Here's how the part is built. I have some questions about the finished solid (model axes, mm). Coordinates: 2 decimals unless noted, no trailing zeros. Order: outer loops, then holes, each group sorted by start corner. A loop starts at its lowest first (then second) coordinate and runs counter-clockwise, first axis right, second up. Notation, with made-up numbers: (-12, 14.25) - (-6, 14.25) arc R31 ccw to (-6, 43.25) - close; hole circle Ø5 at (75.5, 64). An arc over 180 degrees is marked (long way). Answer in a Markdown table with one row per item. Add a question column.
Item 1: If I drill on line 1 along Y through (x, z) = (0, 1.2) (1 decimal); line 2 along X through (y, z) = (28.5, 2.6); line 3 along Y through (x, z) = (2.25, 0.85), over which ranges is the centre line in solid material (lowest first)? Write a range as from..to.
Item 2: I want a section at A-A (x = 0). Please give me the cut outline in (y, z) (1 decimal), plus the area to 3 significant figures.
Item 3: Will this pin go through, and if not, where does the flat tip stop? pin 1 Ø1 at (x, z) = (-3.5, 2) entering from -Y.
Item 4: I want a section at D-D (y = 80). Please give me the cut outline in (x, z) (3 decimals), plus the area to 3 significant figures.
Item 5: I want a section at C-C (z = 2.65). Please give me the cut outline in (x, y) (1 decimal).
Item 6: I want a section at B-B (y = 52.5). Please give me the cut outline in (x, z) (1 decimal).
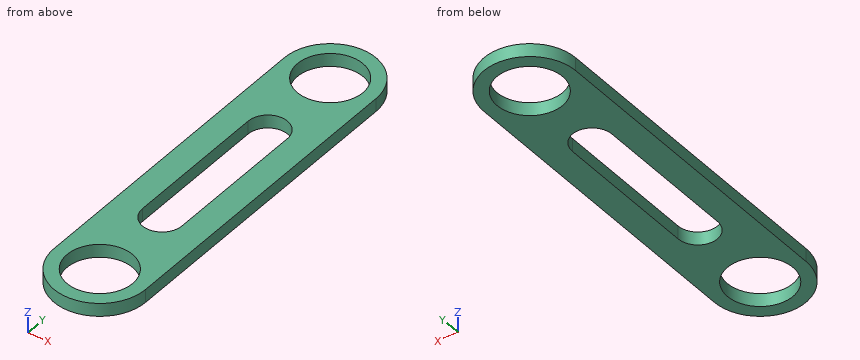
```python
from build123d import *

# Parameters (mm, degrees)
SKETCH1_R           = 7.9375
BOSS_EXTRUDE1_DEPTH = 3.175


with BuildPart() as part:
    # Sketch1 → Boss-Extrude1 (new body)
    with BuildSketch(Plane.XY):
        with BuildLine():
            ThreePointArc((11.1125, 76.2), (0, 87.3125), (-11.1125, 76.2))
            Line((-11.1125, 76.2), (-11.1125, 0))
            ThreePointArc((-11.1125, 0), (0, -11.1125), (11.1125, 0))
            Line((11.1125, 0), (11.1125, 76.2))
        make_face()
        with Locations((0, 76.2)):
            Circle(SKETCH1_R, mode=Mode.SUBTRACT)
        with BuildLine():
            Line((-4.7625, 20.6375), (-4.7625, 55.5625))
            ThreePointArc((-4.7625, 55.5625), (0, 60.325), (4.7625, 55.5625))
            Line((4.7625, 55.5625), (4.7625, 20.6375))
            ThreePointArc((4.7625, 20.6375), (0, 15.875), (-4.7625, 20.6375))
        make_face(mode=Mode.SUBTRACT)
        Circle(SKETCH1_R, mode=Mode.SUBTRACT)
    extrude(amount=BOSS_EXTRUDE1_DEPTH)


solid = part.part
```
Values follow:
| question | item | result |
|---|---|---|
| 1 | line 1 | y = -11.1..-7.9, 7.9..15.9, 60.3..68.3, 84.1..87.3 |
| 1 | line 2 | x = -11.11..-4.76, 4.76..11.11 |
| 1 | line 3 | y = -10.88..-7.61, 7.61..16.44, 59.76..68.59, 83.81..87.08 |
| 2 | outline | (-11.1, 0) - (-7.9, 0) - (-7.9, 3.2) - (-11.1, 3.2) - close; (7.9, 0) - (15.9, 0) - (15.9, 3.2) - (7.9, 3.2) - close; (60.3, 0) - (68.3, 0) - (68.3, 3.2) - (60.3, 3.2) - close; (84.1, 0) - (87.3, 0) - (87.3, 3.2) - (84.1, 3.2) - close |
| 2 | area | 70.6 mm^2 |
| 3 | pin 1 | stops at y = -10.7 |
| 4 | outline | (-10.443, 0) - (-6.969, 0) - (-6.969, 3.175) - (-10.443, 3.175) - close; (6.969, 0) - (10.443, 0) - (10.443, 3.175) - (6.969, 3.175) - close |
| 4 | area | 22.1 mm^2 |
| 5 | outline | (-11.1, 0) arc R11.1 ccw to (11.1, 0) - (11.1, 76.2) arc R11.1 ccw to (-11.1, 76.2) - close; hole circle Ø15.9 at (0, 0); hole circle Ø15.9 at (0, 76.2); hole (-4.8, 20.6) arc R4.8 ccw to (4.8, 20.6) - (4.8, 55.6) arc R4.8 ccw to (-4.8, 55.6) - close |
| 6 | outline | (-11.1, 0) - (-4.8, 0) - (-4.8, 3.2) - (-11.1, 3.2) - close; (4.8, 0) - (11.1, 0) - (11.1, 3.2) - (4.8, 3.2) - close |
